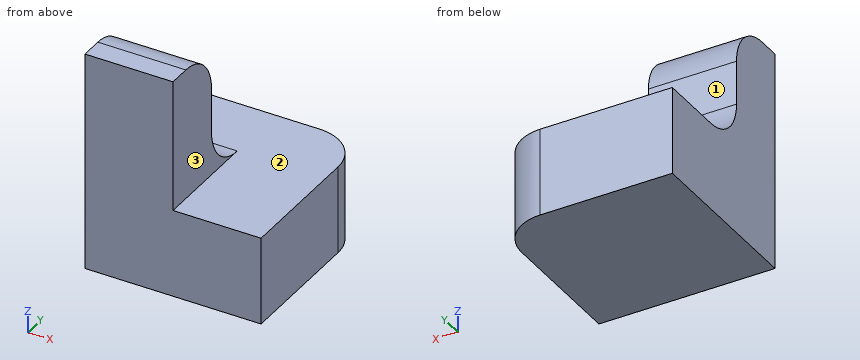
from build123d import *

# Parameters (mm, degrees)
SKETCH1_W           = 20
SKETCH1_H           = 15
BOSS_EXTRUDE1_DEPTH = 30
SKETCH2_W           = 40
SKETCH2_H           = 40
BOSS_EXTRUDE2_DEPTH = 20
FILLET1_R           = 10


with BuildPart() as part:
    # Sketch1 → Boss-Extrude1 (new body)
    with BuildSketch(Plane.XY):
        with Locations((-20, -7.5)):
            Rectangle(SKETCH1_W, SKETCH1_H)
    extrude(amount=BOSS_EXTRUDE1_DEPTH)

    # Sketch2 → Boss-Extrude2 (add)
    with BuildSketch(Plane.XY):
        with Locations((-10, 5)):
            Rectangle(SKETCH2_W, SKETCH2_H)
    extrude(amount=-BOSS_EXTRUDE2_DEPTH)

    # Fillet1
    fillet1_edges = [part.edges().sort_by_distance(p)[0] for p in [
        (10, 25, -10),
        (-20, 0, 30),
        (-20, 0, 0),
    ]]
    fillet(fillet1_edges, radius=FILLET1_R)


solid = part.part
Source: CAD feature listing. Evaluate the final solid. Frame: model axes, mm. Face numbers are marked on the shaded views. A direction names the side the tool comes from. Give positions to 0.01 mm unless a question says otherwise; leave off trailing zeros. Write each loop counter-clockwise with the first axis right and the second up, starting at its lowest first coordinate (ties: lowest second). Pieces come first, ordered by that corner, then holes. Notation, with made-up numbers: (14, -25.5) -> (27, -25.5) arc R15 ccw to (27, -8.5) -> close; hole circle Ø11 at (52.5, -18). An arc over 180 degrees is marked (long way). Return JSON: item names as keys, results as strings. Group by question number.
1. Section D-D, the plane y = -2. Output: boundary loops of the cut face in (x, z).
2. Material intervals for line 1 (Z direction, x = 8.5, y = -5.5); line 2 (Y direction, x = -25.5, z = 15); line 3 (X direction, y = -10.5, z = 23.5), sorted ascending. Write a range as from..to.
3. Section C-C, the plane z = 1. Output: boundary loops of the cut face in (x, y).
4. Section B-B, the plane y = 2. Output: boundary loops of the cut face in (x, z), then the cut area to 3 significant figures.
5. Section A-A, the plane x = -11.5. Output: boundary loops of the cut face in (y, z), then the cut area to 3 significant figures.
6. Access query for the marked faces 1, 2 and 3. Directions: +Z, -Z, +X, -X, +Y, -Y. A direction counts if a zero-diameter tool reaches every point of the face in a straight line with its end or side. Return the directions, or none.
7. Pin query (flat end, axial travel): pin 1 Ø7.5 at (y, z) = (0, 10.5) entering from +X; pin 2 Ø8 at (x, y) = (-1.5, -0.5) entering from +Z; pin 3 Ø11 at (x, z) = (-15.5, 16.5) entering from +Y. Return the tip coordinate at first contact, or that it passes through.
Determined:
{
 "1": {"outline": "(-30, -20) -> (10, -20) -> (10, 0) -> (-10, 0) -> (-10, 26) -> (-30, 26) -> close"},
 "2": {"line 1": "z = -20..0", "line 2": "y = -15..0", "line 3": "x = -30..-10"},
 "3": {"outline": "(-30, -15) -> (-10, -15) -> (-10, 5.64) -> (-30, 5.64) -> close"},
 "4": {"outline": "(-30, -20) -> (10, -20) -> (10, 0) -> (-10, 0) -> (-10, 4) -> (-30, 4) -> close", "area": "880 mm2"},
 "5": {"outline": "(-15, -20) -> (25, -20) -> (25, 0) -> (10, 0) arc R10 cw to (0, 10) -> (0, 20) arc R10 ccw to (-10, 30) -> (-15, 30) -> close", "area": "1,250 mm2"},
 "6": {"face 1": "+Z, +X, -X, +Y", "face 2": "+Z, +X, +Y", "face 3": "+Z, +X, +Y, -Y"},
 "7": {"pin 1": "stops at x = -10", "pin 2": "stops at z = 0", "pin 3": "stops at y = 0"}
}
